For this review, take the finished solid that the model builds, in its own axes (mm). A direction names the side the tool comes from. Coordinates: 2 decimals unless noted, no trailing zeros. Write each loop counter-clockwise with the first axis right and the second up, starting at its lowest first coordinate (ties: lowest second). Pieces come first, ordered by that corner, then holes.
Autodesk Inventor part; units mm, degrees
ref_plane "YZ Plane" through (0, 0, 0) normal (1, 0, 0) x (0, 1, 0)
ref_plane "XZ Plane" through (0, 0, 0) normal (0, 1, 0) x (-1, 0, 0)
ref_plane "XY Plane" through (0, 0, 0) normal (0, 0, 1) x (1, 0, 0)
sketch "Sketch7" plane through (0, 0, 0) normal (0, 1, 0) x (-1, 0, 0)
  line L0 (0, 0) -> (0, -7.9375)
  circle A0 centre (0, -7.9375) radius 1.524
  circle A1 centre (0, 0) radius 3
  circle A2 centre (6.8741, 3.9687) radius 1.524
  circle A3 centre (-6.8741, 3.9688) radius 1.524
  circle A4 centre (0, 0) radius 10.795
  dimension "d32" = 7.9375
  dimension "d33" = 3.048
  dimension "d34" = 6
  dimension "d37" = 360
  dimension "d39" = 21.59
extrude "Extrusion6" add sketch "Sketch7" along normal blind 2.5
sketch "Sketch8" plane through (0, 2.5, 0) normal (0, 1, 0) x (1, 0, 0)
  circle A0 centre (0, 0) radius 4.5
  circle A1 centre (0, 0) radius 6
  dimension "d42" = 9
  dimension "d43" = 12
extrude "Extrusion7" add sketch "Sketch8" along normal blind 1.5
sketch "Sketch9" plane through (0, 2.5, 0) normal (0, 1, 0) x (1, 0, 0)
  circle A0 centre (0, 7.9375) radius 1.524
  circle A1 centre (0, 7.9375) radius 2.8575
  circle A2 centre (-6.8741, -3.9687) radius 2.8575
  circle A3 centre (6.8741, -3.9688) radius 2.8575
  point P0 (0, 0)
  dimension "d46" = 5.715
  dimension "d49" = 360
extrude "Extrusion8" cut sketch "Sketch9" along normal blind 1.5
sketch "Sketch10" plane through (0, 2.5, 0) normal (0, 1, 0) x (1, 0, 0)
  line L0 (0, 0) -> (16.4978, 9.525)
  line L1 (0, 0) -> (19.05, 0) construction
  circle A0 centre (16.4978, 9.525) radius 13.05
  circle A1 centre (-16.4978, 9.525) radius 13.05
  circle A2 centre (0, -19.05) radius 13.05
  dimension "d53" = 19.05
  dimension "d54" = 30
  dimension "d57" = 360
extrude "Extrusion9" cut sketch "Sketch10" against normal through all
fillet "Fillet1" radius 3.175 6 edges at (-3.4665, 1.25, -10.2233) (-10.5869, 1.25, 2.1096) (3.4665, 1.25, -10.2233) (10.5869, 1.25, 2.1096) (7.1204, 1.25, 8.1137) (-7.1204, 1.25, 8.1137)
properties part number "bearingHousing" material "ABS Plastic"
Q1. For probe 1 along X at (y, z) = (1.1, 3.5); probe 2 along Y at (x, z) = (-1.75, -8.5); probe 3 along X at (y, z) = (1.9, -2), list the stretches that pass through material, from the lowest coordinate up.
Ans:
probe 1: x = -9.96 to -8.32, -5.42 to 5.42, 8.32 to 9.96
probe 2: y = 0 to 2.5
probe 3: x = -5.84 to -2.24, 2.24 to 5.84
Q2. Add section B-B (z = -2). State the section outline as (x, y) points, then the cut area to 3 significant figures.
Ans:
outline: (-5.84, 0) - (-2.24, 0) - (-2.24, 2.5) - (-4.03, 2.5) - (-4.03, 4) - (-5.66, 4) - (-5.66, 2.5) - (-5.84, 2.5) - close; (2.24, 0) - (5.84, 0) - (5.84, 2.5) - (5.66, 2.5) - (5.66, 4) - (4.03, 4) - (4.03, 2.5) - (2.24, 2.5) - close
area: 22.9 mm2
Q3. Add section C-C (y = 1.85). Give the number of separate pieces and of enclosed holes in the cut face, then the cut area to 3 significant figures.
Ans:
separate pieces: 1
enclosed holes: 4
area: 168 mm2
Q4. Tool access review of faces 1 (the cylindrical face through (4.39, 3.24, 2.56)), 2 (the cylindrical face through (-4.41, 3.24, 2.52)), 3 (the cylindrical face through (0.03, 3.24, -5.08)), 4 (the flat face through (-4.4, 2.5, 3)): name each direction out of +Z, -Z, +X, -X, +Y, -Y from which nothing blocks a thin tool from reaching the whole face with its end or side.
Ans:
face 1: +X, +Y
face 2: -X, +Y
face 3: -Z, +Y
face 4: +Y
Q5. Add section A-A (z = 0.25). State the section outline as (x, y) points, then the cut area to 3 significant figures.
Ans:
outline: (-7.85, 0) - (-2.99, 0) - (-2.99, 2.5) - (-4.49, 2.5) - (-4.49, 4) - (-5.99, 4) - (-5.99, 2.5) - (-7.85, 2.5) - close; (2.99, 0) - (7.85, 0) - (7.85, 2.5) - (5.99, 2.5) - (5.99, 4) - (4.49, 4) - (4.49, 2.5) - (2.99, 2.5) - close
area: 28.8 mm2
Q6. Draft analysis for pull direction X (two halves, no side actions). For faces 5 (the cylindrical face through (0, 3, 6)), 6 (the cylindrical face through (-9.345, 1.232, 5.404)), 7 (the flat face through (-1, 2.5, -3)), state which applies: +X half, -X half, draft (parallel to the pull), parting line (faces both ways), or undercut.
Ans:
face 5: parting line
face 6: -X half
face 7: undercut
Q7. Clearance check with flat-ended pins moving along their axes: pin 1 Ø5 at (x, z) = (0, 0) entering from -Y; pin 2 Ø1.5 at (x, z) = (-7, -0.5) entering from +Y. State where each tip first meets the part, or that it passes through.
Ans:
pin 1: passes through
pin 2: stops at y = 2.5
